Autodesk Inventor part; units mm, degrees
ref_plane "YZ Plane" through (0, 0, 0) normal (1, 0, 0) x (0, 1, 0)
ref_plane "XZ Plane" through (0, 0, 0) normal (0, 1, 0) x (-1, 0, 0)
ref_plane "XY Plane" through (0, 0, 0) normal (0, 0, 1) x (1, 0, 0)
sketch "Boceto1" plane through (0, 0, 0) normal (0, 0, 1) x (1, 0, 0)
  circle A0 centre (0, 0) radius 1.5
  line L0 (0, 0) -> (28.5, 0)
  line L1 (28.5, 0) -> (28.5, -30)
  circle A1 centre (28.5, -30) radius 1.5
  line L2 (28.5, -30) -> (28.5, -93)
  line L3 (28.5, -93) -> (31, -93)
  circle A2 centre (31, -93) radius 1.5
  line L4 (31, -93) -> (-30, -93)
  circle A3 centre (-30, -93) radius 1.5
  line L5 (-30, -98) -> (31, -98)
  line L6 (31, -98) -> (36, -98)
  line L7 (36, -98) -> (36, 0)
  line L8 (36, 0) -> (36, 5)
  line L9 (36, 5) -> (-30, 5)
  line L10 (-30, 5) -> (-35, 5)
  line L11 (-35, 5) -> (-35, -98)
  line L12 (-35, -98) -> (-30, -98)
  line L13 (-40.5, -46.5) -> (-40.5, -34.5)
  line L14 (-40.5, -46.5) -> (-40.5, -58.5)
  circle A4 centre (-40.5, -34.5) radius 1.5
  circle A5 centre (-40.5, -58.5) radius 1.5
  line L15 (-40.5, -58.5) -> (-77.5, -58.5)
  circle A6 centre (-77.5, -58.5) radius 1.5
  line L16 (-82.5, -58.5) -> (-82.5, -63.5)
  line L17 (-82.5, -63.5) -> (-35, -63.5)
  line L18 (-82.5, -58.5) -> (-82.5, -34.5)
  line L19 (-82.5, -34.5) -> (-82.5, -29.5)
  line L20 (-82.5, -29.5) -> (-38, -29.5)
  line L21 (-38, -29.5) -> (-35, -29.5)
  line L22 (-60.25, -58.5) -> (-77.5, -58.5)
  dimension "d0" = 3
  dimension "d1" = 28.5
  dimension "d2" = 30
  dimension "d3" = 3
  dimension "d4" = 63
  dimension "d5" = 2.5
  dimension "d6" = 3
  dimension "d7" = 61
  dimension "d8" = 3
  dimension "d9" = 5
  dimension "d10" = 5
  dimension "d11" = 5
  dimension "d12" = 5
  dimension "d15" = 12
  dimension "d16" = 12
  dimension "d17" = 3
  dimension "d18" = 3
  dimension "d19" = 37
  dimension "d20" = 3
  dimension "d21" = 5
  dimension "d22" = 5
  dimension "d23" = 5
extrude "Extrusión1" add sketch "Boceto1" along normal blind 5
sketch "Boceto2" plane through (0, 0, 0) normal (0, 0, -1) x (-1, 0, 0)
  circle A0 centre (0, 0) radius 1.5
  circle A1 centre (0, 0) radius 3
  circle A2 centre (-28.5, -30) radius 1.5
  circle A3 centre (-28.5, -30) radius 3
  circle A4 centre (-31, -93) radius 1.5
  circle A5 centre (-31, -93) radius 3
  circle A6 centre (30, -93) radius 1.5
  circle A7 centre (30, -93) radius 3
  circle A8 centre (40.5, -58.5) radius 1.5
  circle A9 centre (40.5, -58.5) radius 3
  circle A10 centre (77.5, -58.5) radius 1.5
  circle A11 centre (77.5, -58.5) radius 3
  circle A12 centre (40.5, -34.5) radius 1.5
  circle A13 centre (40.5, -34.5) radius 3
  dimension "d28" = 6
  dimension "d29" = 6
  dimension "d30" = 6
  dimension "d31" = 6
  dimension "d32" = 6
  dimension "d33" = 6
extrude "Extrusión2" cut sketch "Boceto2" against normal blind 3
sketch "Boceto3" plane through (0, 0, 0) normal (0, 0, -1) x (-1, 0, 0)
  circle A0 centre (-28.5, -30) radius 1.5
  line L0 (-28.5, -30) -> (-21, -30)
  circle A1 centre (0, 0) radius 1.5
  line L1 (0, 0) -> (0, -5)
  circle A2 centre (30, -93) radius 1.5
  line L2 (30, -93) -> (25, -93)
  circle A3 centre (-31, -93) radius 1.5
  line L3 (-31, -93) -> (-24.75, -93)
  line L4 (-24.75, -93) -> (-21, -93)
  circle A4 centre (40.5, -34.5) radius 1.5
  line L5 (40.5, -34.5) -> (40.5, -39.5)
  line L6 (40.5, -34.5) -> (45.5, -34.5)
  circle A5 centre (40.5, -58.5) radius 3
  line L7 (40.5, -58.5) -> (45.5, -58.5)
  circle A6 centre (77.5, -58.5) radius 1.5
  line L8 (77.5, -58.5) -> (77.5, -53.5)
  line L9 (77.5, -53.5) -> (45.5, -34.5)
  line L10 (45.5, -34.5) -> (77.5, -34.5)
  line L11 (77.5, -34.5) -> (77.5, -53.5)
  line L12 (77.5, -58.5) -> (72.5, -58.5)
  line L13 (72.5, -58.5) -> (45.5, -58.5)
  line L14 (40.5, -39.5) -> (72.5, -58.5)
  line L15 (45.5, -58.5) -> (40.5, -39.5)
  line L16 (45.5, -58.5) -> (72.5, -58.5)
  line L17 (59, -58.5) -> (43, -49)
  line L18 (25, -49) -> (2, -5)
  line L19 (-21, -5) -> (-9.5, -27)
  line L20 (13.5, -49) -> (2, -27)
  line L21 (-10.5, -5) -> (2, -27)
  line L22 (-9.5, -49) -> (-21, -27)
  line L23 (25, -27) -> (12.5, -5)
  line L24 (12.5, -5) -> (25, -5)
  line L25 (25, -27) -> (25, -5)
  line L26 (13.5, -49) -> (25, -49)
  line L27 (-21, -27) -> (-9.5, -49)
  line L28 (-21, -27) -> (-21, -5)
  line L29 (-21, -93) -> (-21, -71)
  line L30 (13.5, -93) -> (-9.5, -49)
  line L31 (25, -71) -> (13.5, -49)
  line L32 (-21, -71.6828) -> (-21, -93)
  line L33 (-21, -71.6828) -> (-9.5, -93)
  line L34 (-9.5, -93) -> (-21, -93)
  line L35 (-21, -49) -> (-9.5, -49)
  line L36 (-9.5, -49) -> (13.5, -93)
  line L37 (13.5, -93) -> (2, -93)
  line L38 (25, -71) -> (25, -93)
  line L39 (2, -49) -> (25, -93)
  line L40 (-9.5, -27) -> (2, -49)
  line L41 (2, -49) -> (-9.5, -49)
  line L42 (-21, -27) -> (-21, -5)
  line L43 (-21, -49) -> (-9.5, -49)
  line L44 (-21, -49) -> (2, -93)
  line L45 (2, -93) -> (13.5, -93)
  line L46 (-9.5, -49) -> (13.5, -93)
  line L47 (2, -5) -> (0, -5)
  line L48 (-10.5, -5) -> (0, -5)
  line L49 (2, -49) -> (13.5, -49)
  line L50 (12.5, -5) -> (25, -27)
  line L51 (25, -27) -> (25, -5)
  line L52 (25, -5) -> (12.5, -5)
  line L53 (-21, -27) -> (-21, -5)
  line L54 (-21, -27) -> (-21, -5)
  line L55 (-21, -5) -> (2, -49)
  line L56 (2, -49) -> (-9.5, -49)
  line L57 (-9.5, -49) -> (-21, -27)
  dimension "d36" = 7.5
  dimension "d37" = 5
  dimension "d38" = 5
  dimension "d39" = 5
  dimension "d40" = 5
  dimension "d41" = 5
  dimension "d42" = 5
extrude "Extrusión3" cut sketch "Boceto3" against normal blind 5 contours L10 L11 L9 | L14 L13 L17 L15 | L17 L13 L15 | L26 L20 L21 L48 L47 L18 | L30 L37 L44 L35 | L41 L22 L28 L19 L40 | L31 L38 L39 L49 | L23 L24 L25 | L29 L33 L34
fillet "Empalme1" radius 2 6 edges at (36, -98, 2.5) (-35, -98, 2.5) (-82.5, -63.5, 2.5) (-82.5, -29.5, 2.5) (-35, 5, 2.5) (36, 5, 2.5)
fillet "Empalme2" radius 2 2 edges at (-35, -63.5, 2.5) (-35, -29.5, 2.5)
sketch "Boceto4" plane through (0, 0, 0) normal (0, 0, -1) x (-1, 0, 0)
  line L0 (2, -49) -> (-21, -5)
  line L1 (12.5, -5) -> (25, -5)
  line L2 (-21, -5) -> (25, -5)
  line L3 (25, -93) -> (2, -49)
  line L4 (25, -5) -> (25, -93)
  line L5 (25, -93) -> (-21, -93)
  line L6 (-21, -93) -> (-21, -5)
  point P0 (0, 0)
extrude "Extrusión4" cut sketch "Boceto4" against normal blind 5
sketch "Boceto5" plane through (0, 0, 0) normal (0, 0, -1) x (-1, 0, 0)
  line L0 (-21, -5) -> (-21, -15)
  line L1 (-21, -5) -> (-11, -5)
  line L2 (25, -93) -> (15, -93)
  line L3 (15, -93) -> (-21, -15)
  line L4 (25, -93) -> (25, -83)
  line L5 (25, -83) -> (-11, -5)
  line L6 (-21, -93) -> (-21, -83)
  line L7 (-21, -93) -> (-11, -93)
  line L8 (25, -5) -> (15, -5)
  line L9 (25, -5) -> (25, -15)
  line L10 (25, -15) -> (-11, -93)
  line L11 (15, -5) -> (-21, -83)
  point P0 (0, 0)
  dimension "d49" = 10
  dimension "d50" = 10
  dimension "d51" = 10
  dimension "d52" = 10
  dimension "d53" = 10
  dimension "d54" = 10
  dimension "d55" = 10
  dimension "d56" = 10
extrude "Extrusión5" add sketch "Boceto5" against normal blind 5
properties part number "soporte_nuc_up"
The model under review builds one solid part; all positions refer to its coordinate system, in mm. A direction names the side the tool comes from. Give positions to 0.01 mm unless a question says otherwise; leave off trailing zeros. Write each loop counter-clockwise with the first axis right and the second up, starting at its lowest first coordinate (ties: lowest second). Pieces come first, ordered by that corner, then holes.
1. Wall thickness on L1, parallel to X at y = -16.5, z = 2.3; L2, parallel to Y at x = -58, z = 2.7; L3, parallel to Y at x = -56, z = 4.7: over which ranges is each line inside the solid? List them lowest first.
2. Add section B-B, the plane y = 0. Write out the cut boundary in (x, z).
3. Tool access review of faces 4 (the flat face through (2, -46, 0)), 5 (the flat face through (13.044, -32.238, 2.465)), 6 (the cylindrical face through (3, 0, 1)), 7 (the flat face through (-35, -12, 2)): name each direction out of +Z, -Z, +X, -X, +Y, -Y from which nothing blocks a thin tool from reaching the whole face with its end or side.
4. Add section C-C, the plane x = -7. Write out the cut boundary in (y, z).
5. Draft analysis for pull direction Y (two halves, no side actions). For faces 1 (the cylindrical face through (-75.29, -56.47, 1.48)), 2 (the flat face through (2, -46, 5)), 3 (the flat face through (-59, -63.5, 2)), state which applies: +Y half, -Y half, draft (parallel to the pull), parting line (faces both ways), or undercut.
6. Add section A-A, the plane x = -30. Write out the cut boundary in (y, z).
7. Add section D-D, the plane z = 4.1. Count the separate pieces of the cut face and the enclosed holes in it, plus the area to 3 significant figures.
8. For P1, Ø2.5, axis at x = 0, y = 0, coming from the +Z side; P2, Ø1.5, axis at y = -29.5, z = 0.5, coming from the -X side; P3, Ø2, axis at x = -42, z = 1.5, coming from the -Y side; P4, Ø3, axis at x = -41, y = -35.5, coming from the -Z side, all flat-tipped, find the tip position at first contact; note any pin that passes through.
Worked answers:
1. L1: x = -35 to -25, -24.31 to -9.69, 5.69 to 20.31, 21 to 36
1. L2: y = -63.5 to -58.5, -49.89 to -41.92, -34.5 to -29.5
1. L3: y = -63.5 to -58.5, -48.7 to -40.73, -34.5 to -29.5
2. outline: (-35, 0) - (-3, 0) - (-3, 3) - (-1.5, 3) - (-1.5, 5) - (-35, 5) - close; (1.5, 3) - (3, 3) - (3, 0) - (36, 0) - (36, 5) - (1.5, 5) - close
3. face 4: -Z, +X, -X, +Y, -Y
3. face 5: +Z, -Z
3. face 6: -Z
3. face 7: +Z, -Z, -X, +Y
4. outline: (-98, 0) - (-93, 0) - (-93, 5) - (-98, 5) - close; (-75.67, 0) - (-22.33, 0) - (-22.33, 5) - (-75.67, 5) - close; (-5, 0) - (5, 0) - (5, 5) - (-5, 5) - close
5. face 1: undercut
5. face 2: draft
5. face 3: -Y half
6. outline: (-98, 0) - (-96, 0) - (-96, 3) - (-94.5, 3) - (-94.5, 5) - (-98, 5) - close; (-91.5, 3) - (-90, 3) - (-90, 0) - (5, 0) - (5, 5) - (-91.5, 5) - close
7. separate pieces: 1
7. enclosed holes: 13
7. area: 6,520 mm2
8. P1: passes through
8. P2: stops at x = -82.06
8. P3: stops at y = -63.5
8. P4: stops at z = 3
